Here's how the part is built. I have some questions about the finished solid (model axes, mm). Face numbers are marked on the shaded views. Round coordinates to 2 decimals unless told otherwise and drop trailing zeros. Loops run counter-clockwise (first coordinate to the right, second up) from the corner with the lowest first, then second, coordinate; pieces in that order, holes last. Notation, with made-up numbers: M 2,56.25 L 46,56.25 A17 cw 46,68.25 Z; hole C 2.25,13.25 d4. An arc over 180 degrees is marked long. Answer as a JSON object with one key per item and string values.
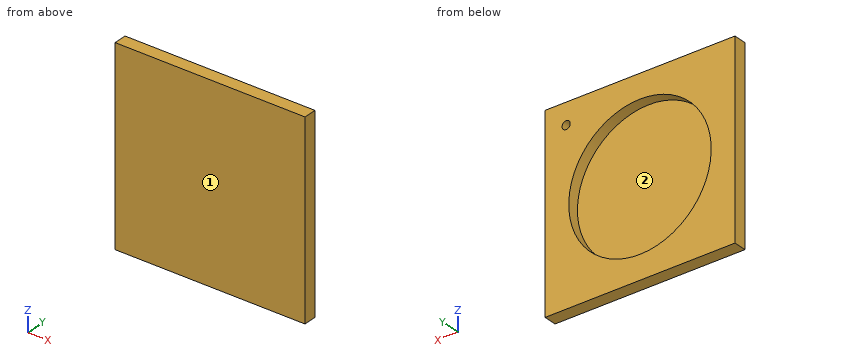
Autodesk Fusion 360 part; units mm, degrees
sketch "Sketch1" plane through (0, 0, 0) normal (0, 1, 0) x (1, 0, 0)
  line L0 (110, 110) -> (-110, 110)
  line L1 (-110, 110) -> (-110, -110)
  line L2 (-110, -110) -> (110, -110)
  line L3 (110, -110) -> (110, 110)
  line L4 (110, 110) -> (-110, -110) construction
  line L5 (-110, 110) -> (110, -110) construction
  circle A0 centre (0, 0) radius 82.5
  circle A1 centre (-85.5, -85.5) radius 15
  circle A2 centre (85.5, -85.5) radius 15
  circle A3 centre (85.5, 85.5) radius 15
  circle A4 centre (-85.5, 85.5) radius 15
  line L6 (0, -110) -> (0, 0) construction
  line L7 (-20, -110) -> (-20, -80.0391)
  line L8 (20, -110) -> (20, -80.0391)
  point P0 (-85.5, -85.5)
  point P1 (85.5, -85.5)
  point P2 (85.5, 85.5)
  point P3 (-85.5, 85.5)
  dimension "d1" = 220
  dimension "d2" = 220
  dimension "d3" = 24.5
  dimension "d4" = 24.5
  dimension "d6" = 360
  dimension "d11" = 165
  dimension "d13" = 30
  dimension "d15" = 360
  dimension "d41" = 20
extrude "Extrude1" add sketch "Sketch1" along normal blind 2 contours L0 L1 L2 L3 A0 L7 L8 | L2 A0 L7 L8 | A0 | A1 | A2 | A3 | A4
sketch "Sketch2" plane through (0, 2, 0) normal (0, 1, 0) x (-1, 0, 0)
  line L0 (-110, 110) -> (-110, -110)
  line L1 (-110, -110) -> (110, -110)
  line L2 (110, -110) -> (110, 110)
  line L3 (110, 110) -> (-110, 110)
  point P0 (85.5, 85.5)
extrude "Extrude2" add sketch "Sketch1" along normal blind 13 from surface at 2 contours L0 L1 L2 L3 A0 L7 L8 | A2 | A3 | A4
sketch "Sketch3" plane through (0, 15, 0) normal (0, 1, 0) x (-1, 0, 0)
  line L0 (110, 110) -> (20, 110)
  line L1 (-110, 110) -> (-110, -110)
  line L2 (-110, -110) -> (110, -110)
  line L3 (110, -110) -> (110, 110)
  circle A0 centre (85.5, 85.5) radius 15
  line L4 (20, 110) -> (20, 80.0391)
  arc A1 (-20, 80.0391) -> (20, 80.0391) centre (0, 0) ccw
  line L5 (-20, 80.0391) -> (-20, 110)
  line L6 (-20, 110) -> (-110, 110)
  point P0 (85.5, -85.5)
  point P1 (-85.5, -85.5)
  point P2 (85.5, 85.5)
  point P3 (-85.5, 85.5)
hole "Hole3" at (-85.5, 15, -85.5) at (85.5, 15, -85.5) at (-85.5, 15, 85.5) at (85.5, 15, 85.5) direction (0, -1, 0) diameter 4.5 depth 15 tip angle 180
hole "Hole5" at (-85.5, 15, -85.5) at (-85.5, 15, 85.5) at (85.5, 15, 85.5) at (85.5, 15, -85.5) direction (0, -1, 0) diameter 9.4 depth 13 tip angle 118
pattern_circular "C-Pattern1" count 2 over 90 about axis through (0, 1.75, 0) along (0, 1, 0) of "Extrude1", "Extrude2"
equation "overall_height = 15 mm"
equation "cutout_depth = 13 mm"
equation "wafer_slot_diameter = 165 mm"
equation "cuevette_slot_diam = 30 mm"
equation "d11 = wafer_slot_diameter"
equation "screw_plate_thickness = 2 mm"
equation "d13 = cuevette_slot_diam"
equation "d16 = screw_plate_thickness"
equation "d18 = overall_height - screw_plate_thickness"
equation "d20 = screw_plate_thickness"
equation "d42 = overall_height - screw_plate_thickness"
Item 1: I want a section at C-C on y = 7.75. List the corners of the cut face in (x, z) for me.
Solution:
{"outline": "M -110,-110 L 110,-110 L 110,110 L -110,110 Z; hole C 0,0 d165; hole C 85.5,85.5 d9.4"}
Item 2: If I drill on L1, parallel to Z at x = 0, y = 5; L2, parallel to X at y = 8, z = 85.5, over which ranges is the centre line in solid material (lowest first)? Write a range as from..to.
Solution:
{"L1": "z = -110..-82.5, 82.5..110", "L2": "x = -110..80.8, 90.2..110"}
Item 3: We'd pull the mould along X, two halves only. Please class the marked faces 1 and 2: +X half, -X half, draft (parallel to the pull), parting line (faces both ways), or undercut.
Solution:
{"face 1": "draft", "face 2": "undercut"}
Item 4: I want a section at A-A on z = 0. List the corners of the cut face in (x, y) for me, plus the area to 4 significant figures.
Solution:
{"outline": "M -110,0 L 110,0 L 110,15 L 82.5,15 L 82.5,2 L -82.5,2 L -82.5,15 L -110,15 Z", "area": "1,155 mm2"}
Item 5: For P1, Ø10, axis at x = -28, z = -61.5, coming from the +Y side, with a flat end and sliding along its axis, tell me the tip position at first contact or that it passes through.
Solution:
{"P1": "stops at y = 2"}
Item 6: I want a section at B-B on x = 0. List the corners of the cut face in (y, z) for me.
Solution:
{"outline": "M 0,-110 L 15,-110 L 15,-82.5 L 2,-82.5 L 2,82.5 L 15,82.5 L 15,110 L 0,110 Z"}
